For this review, take the finished solid that the model builds, in its own axes (mm). Face numbers are marked on the shaded views. A direction names the side the tool comes from. Give positions to 0.01 mm unless a question says otherwise; leave off trailing zeros. Order: outer loops, then holes, each group sorted by start corner. A loop starts at its lowest first (then second) coordinate and runs counter-clockwise, first axis right, second up. Notation, with made-up numbers: (40, 73.5) - (80, 73.5) arc R37 cw to (80, 112.5) - close; hole circle Ø8 at (65, 72). An arc over 180 degrees is marked (long way). Put each result on its own line as item: value. Start each with the question number.
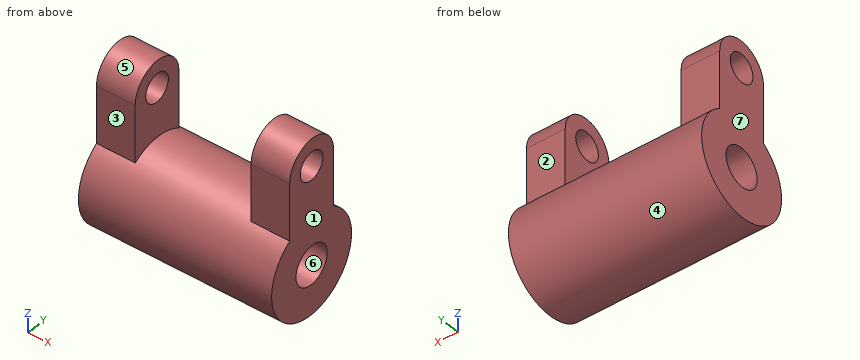
```python
from build123d import *

# Parameters (mm, degrees)
F0_R      = 33.0702193876
F1_DEPTH  = 63.5
F3_DEPTH  = 25.4
F7_DEPTH  = 25.4
F8_DEPTH  = 25.4
F9_R      = 12.915127355
F10_DEPTH = 127.001
F11_R     = 9.381167956
F12_DEPTH = 127.001


with BuildPart() as f1:
    # F0 (on Right) → F1 (new body)
    with BuildSketch(Plane.YZ):
        Circle(F0_R)
    extrude(amount=-F1_DEPTH)

    # F2 (on face) → F3 (join)
    with BuildSketch(Plane.YZ):
        with BuildLine():
            Line((-18.0798303336, 66.1404387753), (-18.0798303336, 27.69041613))
            ThreePointArc((-18.0798303336, 27.69041613), (0, 33.0702193876), (18.0798303336, 27.69041613))
            Line((18.0798303336, 27.69041613), (18.0798303336, 66.1404387753))
            Line((18.0798303336, 66.1404387753), (-18.0798303336, 66.1404387753))
        make_face()
        with BuildLine():
            Line((-18.0798303336, 27.69041613), (-18.0798303336, 0))
            Line((-18.0798303336, 0), (18.0798303336, 0))
            Line((18.0798303336, 0), (18.0798303336, 27.69041613))
            ThreePointArc((18.0798303336, 27.69041613), (0, 33.0702193876), (-18.0798303336, 27.69041613))
        make_face()
    extrude(amount=-F3_DEPTH)

    # F4: F1 across face


with BuildPart() as f1_1:
    add(f1.part)
    add(f1.part.mirror(Plane(origin=(-63.5, 0, 0), x_dir=(0, 1, 0), z_dir=(-1, 0, 0))))

    # F5 (on face) → F7 (join)
    with BuildSketch(Plane.YZ):
        with BuildLine():
            ThreePointArc((-18.0798303336, 66.1404387753), (0, 48.0606084417), (18.0798303336, 66.1404387753))
            Line((18.0798303336, 66.1404387753), (-18.0798303336, 66.1404387753))
        make_face()
        with BuildLine():
            Line((-18.0798303336, 66.1404387753), (18.0798303336, 66.1404387753))
            ThreePointArc((18.0798303336, 66.1404387753), (0, 84.2202691088), (-18.0798303336, 66.1404387753))
        make_face()
    extrude(amount=-F7_DEPTH)

    # F6 (on face) → F8 (join)
    with BuildSketch(Plane(origin=(-127, 0, 0), x_dir=(0, -1, 0), z_dir=(-1, 0, 0))):
        with BuildLine():
            Line((-18.0798303336, 66.1404387753), (18.0798303336, 66.1404387753))
            ThreePointArc((18.0798303336, 66.1404387753), (0, 84.2202691088), (-18.0798303336, 66.1404387753))
        make_face()
    extrude(amount=-F8_DEPTH)

    # F9 (on face) → F10 (cut, through all)
    with BuildSketch(Plane(origin=(-127, 0, 0), x_dir=(0, -1, 0), z_dir=(-1, 0, 0))):
        Circle(F9_R)
    extrude(amount=-F10_DEPTH, mode=Mode.SUBTRACT)

    # F11 (on face) → F12 (cut, through all)
    with BuildSketch(Plane.YZ):
        with Locations((0, 66.1404387753)):
            Circle(F11_R)
    extrude(amount=-F12_DEPTH, mode=Mode.SUBTRACT)


solid = f1_1.part
```
1. Add section D-D, the plane z = 0. Give the boundary of the cut face in (x, y).
2. The part is to be moulded in two halves that separate along Z. For the marked faces 4, 5, 6 and 7, say which applies: released by +Z, released by -Z, zero draft, split by the parting line, or undercut.
3. Tool access review of the marked faces 1, 2 and 3: name each direction out of +Z, -Z, +X, -X, +Y, -Y from which nothing blocks a thin tool from reaching the whole face with its end or side.
4. Add section B-B, the plane y = 0. Give the boundary of the cut face in (x, z), then the cut area to 3 significant figures.
5. Add section C-C, the plane x = -8.5. Give the boundary of the cut face in (y, z), then the cut area to 3 significant figures.
6. Wall thickness on line 1 (Z direction, x = -7.25, y = 0); line 2 (X direction, y = -15, z = 40.5); line 3 (Y direction, x = -78.5, z = -5): over which ranges is each line inside the solid? List them lowest first. Write a range as from..to.
7. Add section A-A, the plane z = 49.5. Give the boundary of the cut face in (x, y), then the cut area to 3 significant figures.
8. Clearance check with flat-ended pins moving along their axes: pin 1 (12.5 mm diameter, centred on x = -110, z = 53, fed in from -Y); pin 2 (12 mm diameter, centred on x = -16.5, z = 18, fed in from +Y); pin 3 (1 mm diameter, centred on x = -65, z = 29.5, fed in from -Y). State where each tip first meets the part, or that it passes through.
Found:
1. outline: (-127, -33.07) - (0, -33.07) - (0, -12.92) - (-127, -12.92) - close; (-127, 12.92) - (0, 12.92) - (0, 33.07) - (-127, 33.07) - close
2. face 4: split by the parting line
2. face 5: released by +Z
2. face 6: undercut
2. face 7: zero draft
3. face 1: +Z, -Z, +X, +Y, -Y
3. face 2: +Z, +X, -X, +Y
3. face 3: +Z, +X, -X, -Y
4. outline: (-127, -33.07) - (0, -33.07) - (0, -12.92) - (-127, -12.92) - close; (-127, 12.92) - (0, 12.92) - (0, 56.76) - (-25.4, 56.76) - (-25.4, 33.07) - (-101.6, 33.07) - (-101.6, 56.76) - (-127, 56.76) - close; (-127, 75.52) - (-101.6, 75.52) - (-101.6, 84.22) - (-127, 84.22) - close; (-25.4, 75.52) - (0, 75.52) - (0, 84.22) - (-25.4, 84.22) - close
4. area: 6,760 mm^2
5. outline: (-18.08, 27.69) arc R33.07 ccw (long way) to (18.08, 27.69) - (18.08, 66.14) arc R18.08 ccw to (-18.08, 66.14) - close; hole circle Ø25.83 at (0, 0); hole circle Ø18.76 at (0, 66.14)
5. area: 4,410 mm^2
6. line 1: z = -33.07..-12.92, 12.92..56.76, 75.52..84.22
6. line 2: x = -127..-101.6, -25.4..0
6. line 3: y = -32.69..-11.91, 11.91..32.69
7. outline: (-127, -18.08) - (-101.6, -18.08) - (-101.6, 18.08) - (-127, 18.08) - close; (-25.4, -18.08) - (0, -18.08) - (0, 18.08) - (-25.4, 18.08) - close
7. area: 1,840 mm^2
8. pin 1: stops at y = -18.08
8. pin 2: stops at y = 30.82
8. pin 3: stops at y = -15.89
